Geometry check sheet. Reference: the model listing, model coordinates, mm. A direction names the side the tool comes from. Give positions to 0.01 mm unless a question says otherwise; leave off trailing zeros. Loops run counter-clockwise (first coordinate to the right, second up) from the corner with the lowest first, then second, coordinate; pieces in that order, holes last. Notation, with made-up numbers: (-25, 30.5) -> (1, 30.5) arc R29 ccw to (1, 59.5) -> close; hole circle Ø1 at (-12, 79.25). An arc over 180 degrees is marked (long way). One line per item, written item: value. Start each with the question number.
(1) Tool access check on faces 4 (the face through (69.4, 1.52, -0.57)), 5 (the face through (35, 1, -25)), 6 (the face through (48.15, 1.48, -17.99)). Record the directions out of +Z, -Z, +X, -X, +Y, -Y that give a thin tool (end or side, any length) a straight path to the whole face; none if there is none.
(2) Sectioned sample at A-A, the plane z = -3. Record the cut outline in (x, y), then the cut area to 3 significant figures.
(3) Sectioned sample at D-D, the plane z = -52. Record the cut outline in (x, y), then the cut area to 3 significant figures.
(4) Draft check along Z on faces 1 (the face through (9, 1, 0)), 2 (the face through (51, 2, -6)), 3 (the face through (16.94, 1.48, -41.92)). Enter one of: pulls with the +Z half, pulls with the -Z half, needs draft (parallel to the pull), parting line crosses it, or undercut.
(5) Sectioned sample at C-C, the plane z = -43.5. Record the cut outline in (x, y).
(6) Sectioned sample at B-B, the plane x = 67. Record the cut outline in (y, z).
(7) Gauge pin test, flat ends, axial feed: pin 1 Ø2.5 at (x, z) = (54, -3) entering from +Y; pin 2 Ø12 at (x, z) = (22, -42) entering from -Y. Record the tip position at first contact, or that the pin passes through.
(8) Scan lines: line 1 along X through (y, z) = (2.3, -5); line 2 along X through (y, z) = (1.2, -17.5); line 3 along X through (y, z) = (2.15, -10). Record each from-to range of solid material in increasing order. Write a range as from..to.
from build123d import *

# Parameters (mm, degrees)
SKETCH_1_W          = 70
SKETCH_1_H          = 58
SKETCH_1_R          = 7
EXTRUDE_1_DEPTH     = 3
CHAMFER_1_SIZE      = 20
SKETCH_2_W          = 32
SKETCH_2_H          = 21
CUT_EXTRUDE_1_DEPTH = 3
FILLET_1_R          = 10
SKETCH_3_R          = 1.5
CUT_EXTRUDE_2_DEPTH = 91.956033335
SKETCH_4_R          = 1.5
CUT_EXTRUDE_3_DEPTH = 91.956033335
FILLET_2_R          = 2
SKETCH_5_W          = 14
SKETCH_5_H          = 7
CUT_EXTRUDE_4_DEPTH = 91.956033335
FILLET_3_R          = 3
FILLET_4_R          = 5
SKETCH_6_R          = 3.5
CUT_EXTRUDE_5_DEPTH = 10


with BuildPart() as part:
    # 草图1 → 凸台-拉伸1 (new body)
    with BuildSketch(Plane(origin=(0, 0, 0), x_dir=(1, 0, 0), z_dir=(0, 1, 0))):
        with Locations((35, 29)):
            Rectangle(SKETCH_1_W, SKETCH_1_H)
        with Locations(Location((35, 43.5, 0), (0, 0, 270))):
            Circle(SKETCH_1_R, mode=Mode.SUBTRACT)
    extrude(amount=EXTRUDE_1_DEPTH)

    # 倒角1
    chamfer_1_edges = [part.edges().sort_by_distance(p)[0] for p in [
        (0, 1.5, -58),
        (70, 1.5, -58),
    ]]
    chamfer(chamfer_1_edges, length=CHAMFER_1_SIZE)

    # 草图2 → 切除-拉伸1 (cut)
    with BuildSketch(Plane(origin=(0, 3, 0), x_dir=(1, 0, 0), z_dir=(0, 1, 0))):
        with Locations((35, 10.5)):
            Rectangle(SKETCH_2_W, SKETCH_2_H)
    extrude(amount=-CUT_EXTRUDE_1_DEPTH, mode=Mode.SUBTRACT)

    # 圆角1
    fillet_1_edges = [part.edges().sort_by_distance(p)[0] for p in [
        (51, 1.5, -21),
        (19, 1.5, -21),
    ]]
    fillet(fillet_1_edges, radius=FILLET_1_R)

    # 草图3 → 切除-拉伸2 (cut, through all)
    with BuildSketch(Plane(origin=(0, 3, 0), x_dir=(1, 0, 0), z_dir=(0, 1, 0))):
        with Locations(Location((3, 17, 0), (0, 0, 270))):
            Circle(SKETCH_3_R)
        with Locations(Location((16, 17, 0), (0, 0, 270))):
            Circle(SKETCH_3_R)
        with Locations(Location((3, 3, 0), (0, 0, 270))):
            Circle(SKETCH_3_R)
        with Locations(Location((16, 3, 0), (0, 0, 270))):
            Circle(SKETCH_3_R)
        with Locations(Location((54, 3, 0), (0, 0, 90))):
            Circle(SKETCH_3_R)
        with Locations(Location((67, 3, 0), (0, 0, 90))):
            Circle(SKETCH_3_R)
        with Locations(Location((54, 17, 0), (0, 0, 90))):
            Circle(SKETCH_3_R)
        with Locations(Location((67, 17, 0), (0, 0, 90))):
            Circle(SKETCH_3_R)
    extrude(amount=-CUT_EXTRUDE_2_DEPTH, mode=Mode.SUBTRACT)

    # 草图4 → 切除-拉伸3 (cut, through all)
    with BuildSketch(Plane.XZ):
        with Locations(Location((21.071067812, -52, 0), (0, 0, 270))):
            Circle(SKETCH_4_R)
        with Locations(Location((6, -36.928932188, 0), (0, 0, 270))):
            Circle(SKETCH_4_R)
        with Locations(Location((64, -36.928932188, 0), (0, 0, 90))):
            Circle(SKETCH_4_R)
        with Locations(Location((48.928932188, -52, 0), (0, 0, 90))):
            Circle(SKETCH_4_R)
    extrude(amount=-CUT_EXTRUDE_3_DEPTH, mode=Mode.SUBTRACT)

    # 圆角2
    fillet_2_edges = [part.edges().sort_by_distance(p)[0] for p in [
        (51, 1.5, 0),
        (19, 1.5, 0),
        (70, 1.5, 0),
        (0, 1.5, 0),
    ]]
    fillet(fillet_2_edges, radius=FILLET_2_R)

    # 草图5 → 切除-拉伸4 (cut, through all)
    with BuildSketch(Plane.XZ):
        with BuildLine():
            Line((43.356238926, -33.541422239), (54.283628291, -20.518666706))
            ThreePointArc((54.283628291, -20.518666706), (58.175259711, -24.449873037), (61.27895346, -29.028766292))
            Line((61.27895346, -29.028766292), (57.414380707, -41.538995788))
            Line((57.414380707, -41.538995788), (47.950531075, -42.366975344))
            ThreePointArc((47.950531075, -42.366975344), (46.531140831, -37.497268028), (43.356238926, -33.541422239))
        make_face()
        with BuildLine():
            Line((26.643761074, -33.541422239), (15.716371709, -20.518666706))
            ThreePointArc((15.716371709, -20.518666706), (11.824740289, -24.449873037), (8.72104654, -29.028766292))
            Line((8.72104654, -29.028766292), (12.585619293, -41.538995788))
            Line((12.585619293, -41.538995788), (22.049468925, -42.366975344))
            ThreePointArc((22.049468925, -42.366975344), (23.468859169, -37.497268028), (26.643761074, -33.541422239))
        make_face()
        with Locations((35, -28.5)):
            Rectangle(SKETCH_5_W, SKETCH_5_H)
    extrude(amount=-CUT_EXTRUDE_4_DEPTH, mode=Mode.SUBTRACT)

    # 圆角3
    fillet_3_edges = [part.edges().sort_by_distance(p)[0] for p in [
        (22.049468925, 1.5, -42.366975344),
        (12.585619293, 1.5, -41.538995788),
        (8.72104654, 1.5, -29.028766292),
        (15.716371709, 1.5, -20.518666706),
        (54.283628291, 1.5, -20.518666706),
        (61.27895346, 1.5, -29.028766292),
        (57.414380707, 1.5, -41.538995788),
        (47.950531075, 1.5, -42.366975344),
        (42, 1.5, -25),
        (42, 1.5, -32),
        (28, 1.5, -32),
        (28, 1.5, -25),
    ]]
    fillet(fillet_3_edges, radius=FILLET_3_R)

    # 圆角4
    fillet_4_edges = [part.edges().sort_by_distance(p)[0] for p in [
        (26.643761074, 1.5, -33.541422239),
        (43.356238926, 1.5, -33.541422239),
    ]]
    fillet(fillet_4_edges, radius=FILLET_4_R)

    # 草图6 → 切除-拉伸5 (cut)
    with BuildSketch(Plane.XZ):
        with Locations(Location((9.5, -10, 0), (0, 0, 270))):
            Circle(SKETCH_6_R)
        with Locations(Location((60.5, -10, 0), (0, 0, 270))):
            Circle(SKETCH_6_R)
    extrude(amount=-CUT_EXTRUDE_5_DEPTH, mode=Mode.SUBTRACT)


solid = part.part
Calculated:
1. face 4: +Z, +X, +Y, -Y
1. face 5: +Y, -Y
1. face 6: +Z, +Y, -Y
2. outline: (0, 0) -> (1.5, 0) -> (1.5, 3) -> (0, 3) -> close; (4.5, 0) -> (14.5, 0) -> (14.5, 3) -> (4.5, 3) -> close; (17.5, 0) -> (19, 0) -> (19, 3) -> (17.5, 3) -> close; (51, 0) -> (52.5, 0) -> (52.5, 3) -> (51, 3) -> close; (55.5, 0) -> (65.5, 0) -> (65.5, 3) -> (55.5, 3) -> close; (68.5, 0) -> (70, 0) -> (70, 3) -> (68.5, 3) -> close
2. area: 78.0 mm2
3. outline: (14, 0) -> (19.57, 0) -> (19.57, 3) -> (14, 3) -> close; (22.57, 0) -> (47.43, 0) -> (47.43, 3) -> (22.57, 3) -> close; (50.43, 0) -> (56, 0) -> (56, 3) -> (50.43, 3) -> close
3. area: 108 mm2
4. face 1: pulls with the +Z half
4. face 2: needs draft
4. face 3: undercut
5. outline: (5.5, 0) -> (28, 0) -> (28, 3) -> (5.5, 3) -> close; (42, 0) -> (64.5, 0) -> (64.5, 3) -> (42, 3) -> close
6. outline: (0, -41) -> (3, -41) -> (3, -18.5) -> (0, -18.5) -> close; (0, -15.5) -> (3, -15.5) -> (3, -4.5) -> (0, -4.5) -> close; (0, -1.5) -> (3, -1.5) -> (3, 0) -> (0, 0) -> close
7. pin 1: passes through
7. pin 2: stops at y = 0
8. line 1: x = 0..19, 51..70
8. line 2: x = 0..1.59, 4.41..14.59, 17.41..21.4, 48.6..52.59, 55.41..65.59, 68.41..70
8. line 3: x = 0..6, 13..19, 51..57, 64..70
